```python
from build123d import *

# Parameters (mm, degrees)
SKETCH_1_W          = 600
SKETCH_1_H          = 400
EXTRUDE_1_DEPTH     = 3
SKETCH_3_W          = 100
SKETCH_3_H          = 100
CUT_EXTRUDE_1_DEPTH = 361.567608085
SKETCH_4_R          = 2
CUT_EXTRUDE_2_DEPTH = 361.567608085
SKETCH_5_R          = 1.6
CUT_EXTRUDE_3_DEPTH = 361.567608085
SKETCH_6_R          = 10.05
CUT_EXTRUDE_4_DEPTH = 361.567608085
SKETCH_7_R          = 1.5
CUT_EXTRUDE_5_DEPTH = 361.567608085


with BuildPart() as part:
    # 草图1 → 凸台-拉伸1 (new body)
    with BuildSketch(Plane.XY):
        Rectangle(SKETCH_1_W, SKETCH_1_H)
    extrude(amount=EXTRUDE_1_DEPTH)

    # 草图3 → 切除-拉伸1 (cut, through all)
    with BuildSketch(Plane(origin=(0, 0, 0), x_dir=(-1, 0, 0), z_dir=(0, 0, -1))):
        Rectangle(SKETCH_3_W, SKETCH_3_H)
    extrude(amount=-CUT_EXTRUDE_1_DEPTH, mode=Mode.SUBTRACT)

    # 草图4 → 切除-拉伸2 (cut, through all)
    with BuildSketch(Plane.XY.offset(3)):
        with Locations((-50, 50)):
            Circle(SKETCH_4_R)
        with Locations((-50, -50)):
            Circle(SKETCH_4_R)
        with Locations((50, -50)):
            Circle(SKETCH_4_R)
        with Locations((50, 50)):
            Circle(SKETCH_4_R)
    extrude(amount=-CUT_EXTRUDE_2_DEPTH, mode=Mode.SUBTRACT)

    # 草图5 → 切除-拉伸3 (cut, through all)
    with BuildSketch(Plane(origin=(0, 0, 0), x_dir=(-1, 0, 0), z_dir=(0, 0, -1))):
        with Locations((-297, 169)):
            Circle(SKETCH_5_R)
        with Locations((-297, 189)):
            Circle(SKETCH_5_R)
        with Locations((-279, 197)):
            Circle(SKETCH_5_R)
        with Locations((-259, 197)):
            Circle(SKETCH_5_R)
        with Locations(Location((-259, -197, 0), (0, 0, 180))):
            Circle(SKETCH_5_R)
        with Locations(Location((-279, -197, 0), (0, 0, 180))):
            Circle(SKETCH_5_R)
        with Locations(Location((-297, -189, 0), (0, 0, 180))):
            Circle(SKETCH_5_R)
        with Locations(Location((-297, -169, 0), (0, 0, 180))):
            Circle(SKETCH_5_R)
    extrude(amount=-CUT_EXTRUDE_3_DEPTH, mode=Mode.SUBTRACT)

    # 草图6 → 切除-拉伸4 (cut, through all)
    with BuildSketch(Plane(origin=(0, 0, 0), x_dir=(-1, 0, 0), z_dir=(0, 0, -1))):
        with Locations((0, 100)):
            Circle(SKETCH_6_R)
        with Locations(Location((0, -100, 0), (0, 0, 180))):
            Circle(SKETCH_6_R)
    extrude(amount=-CUT_EXTRUDE_4_DEPTH, mode=Mode.SUBTRACT)

    # 草图7 → 切除-拉伸5 (cut, through all)
    with BuildSketch(Plane(origin=(0, 0, 0), x_dir=(-1, 0, 0), z_dir=(0, 0, -1))):
        with Locations((-297, -56.5)):
            Circle(SKETCH_7_R)
        with Locations((-297, -76.5)):
            Circle(SKETCH_7_R)
        with Locations(Location((-297, 76.5, 0), (0, 0, 180))):
            Circle(SKETCH_7_R)
        with Locations(Location((-297, 56.5, 0), (0, 0, 180))):
            Circle(SKETCH_7_R)
    extrude(amount=-CUT_EXTRUDE_5_DEPTH, mode=Mode.SUBTRACT)


solid = part.part
```
Work out the finished part from the listing and answer in its coordinate system (mm). Give positions to 0.01 mm unless a question says otherwise; leave off trailing zeros. Loops run counter-clockwise (first coordinate to the right, second up) from the corner with the lowest first, then second, coordinate; pieces in that order, holes last. Notation, with made-up numbers: (54, 57) -> (91, 57) arc R36 cw to (91, 94) -> close; hole circle Ø2 at (45, 20.25). An arc over 180 degrees is marked (long way). Write item = value, one per line. Start each with the question number.
(1) Find section A-A on x = -22. Give the vertices of the cut face in (y, z), and give its area (3 significant figures).
(2) The mould has two halves that part along X. Classify faces 1 (the flat face through (-71, 3, 3)), 2 (the cylindrical face through (-7.4, -106.8, 1.5)), 3 (the cylindrical face through (-5.403, 108.474, 1.479)): +X half, -X half, draft (parallel to the pull), parting line (faces both ways), or undercut.
(3) Find section C-C on z = 1. Give the number of separate pieces and of enclosed holes in the cut face, and give its area (3 significant figures).
(4) Find section B-B on y = -8.5. Give the vertices of the cut face in (x, z).
(5) Find the intervals of material crossed by probe 1 along Y at (x, z) = (279, 0.7); probe 2 along X at (y, z) = (-197, 2.4); probe 3 along Y at (x, z) = (-4.5, 1.05), in increasing order. Write a range as from..to.
From the geometry:
q1.outline = (-200, 0) -> (-50, 0) -> (-50, 3) -> (-200, 3) -> close; (50, 0) -> (200, 0) -> (200, 3) -> (50, 3) -> close
q1.area = 900 mm^2
q2.face_1 = draft
q2.face_2 = undercut
q2.face_3 = undercut
q3.separate_pieces = 1
q3.enclosed_holes = 15
q3.area = 229,000 mm^2
q4.outline = (-300, 0) -> (-50, 0) -> (-50, 3) -> (-300, 3) -> close; (50, 0) -> (300, 0) -> (300, 3) -> (50, 3) -> close
q5.probe_1 = -200..-198.6, -195.4..195.4, 198.6..200
q5.probe_2 = -300..257.4, 260.6..277.4, 280.6..300
q5.probe_3 = -200..-108.99, -91.01..-50, 50..91.01, 108.99..200
